```python
from build123d import *

# Parameters (mm, degrees)
SKETCH1_W                      = 260
SKETCH1_H                      = 250
BASE_FLANGE1_DEPTH             = 8
SKETCH2_R                      = 30
CUT_EXTRUDE1_DEPTH             = 10
EDGE_FLANGE1_STRIP_W           = 62
EDGE_FLANGE1_STRIP_H           = 8
EDGE_FLANGE1_STRIP_CUT_DEPTH   = 260
EDGE_FLANGE1_STRIP_2_W         = 62
EDGE_FLANGE1_STRIP_2_H         = 8
EDGE_FLANGE1_STRIP_CUT_2_DEPTH = 260
EDGE_FLANGE1_DEPTH             = 260
EDGE_FLANGE1_BEND_DEPTH        = 260
SKETCH9_R                      = 9
CUT_EXTRUDE2_DEPTH             = 10
SKETCH10_R                     = 8
CUT_EXTRUDE3_DEPTH             = 10
CIRPATTERN1_COUNT              = 4


# Sheet-metal steps are written as plain solids
with BuildPart() as part:
    # Sketch1 → Base-Flange1 (new body)
    with BuildSketch(Plane(origin=(0, 0, 0), x_dir=(0, 0, -1), z_dir=(1, 0, 0))):
        Rectangle(SKETCH1_W, SKETCH1_H)
    extrude(amount=-BASE_FLANGE1_DEPTH)

    # Sketch2 → Cut-Extrude1 (cut)
    with BuildSketch(Plane(origin=(0, 0, 0), x_dir=(0, 0, -1), z_dir=(1, 0, 0))):
        Circle(SKETCH2_R)
    extrude(amount=-CUT_EXTRUDE1_DEPTH, mode=Mode.SUBTRACT)

    # Edge-Flange1 strip (across the edge) → Edge-Flange1 strip cut (cut)
    with BuildSketch(Plane(origin=(0, 125, -130), x_dir=(0, -1, 0), z_dir=(0, 0, 1))):
        with Locations((-8, -4)):
            Rectangle(EDGE_FLANGE1_STRIP_W, EDGE_FLANGE1_STRIP_H)
    extrude(amount=EDGE_FLANGE1_STRIP_CUT_DEPTH, mode=Mode.SUBTRACT)

    # Edge-Flange1 strip 2 (across the edge) → Edge-Flange1 strip cut 2 (cut)
    with BuildSketch(Plane(origin=(0, -125, 130), x_dir=(0, 1, 0), z_dir=(0, 0, -1))):
        with Locations((-8, -4)):
            Rectangle(EDGE_FLANGE1_STRIP_2_W, EDGE_FLANGE1_STRIP_2_H)
    extrude(amount=EDGE_FLANGE1_STRIP_CUT_2_DEPTH, mode=Mode.SUBTRACT)

    # Edge-Flange1 section (across the edge) → Edge-Flange1 (add)
    with BuildSketch(Plane(origin=(0, 125, -130), x_dir=(0, -1, 0), z_dir=(0, 0, 1))):
        with BuildLine():
            Line((0, 15), (0, 32))
            Line((0, 32), (8, 32))
            Line((8, 32), (8, 15))
            ThreePointArc((8, 15), (12.393398282, 4.393398282), (23, 0))
            Line((23, 0), (23, -8))
            ThreePointArc((23, -8), (6.736544033, -1.263455967), (0, 15))
        make_face()
    extrude(amount=EDGE_FLANGE1_DEPTH)

    # Edge-Flange1 section 2 (across the edge) → Edge-Flange1 bend (add)
    with BuildSketch(Plane(origin=(0, -125, 130), x_dir=(0, 1, 0), z_dir=(0, 0, -1))):
        with BuildLine():
            Line((0, 15), (0, 32))
            Line((0, 32), (8, 32))
            Line((8, 32), (8, 15))
            ThreePointArc((8, 15), (12.393398282, 4.393398282), (23, 0))
            Line((23, 0), (23, -8))
            ThreePointArc((23, -8), (6.736544033, -1.263455967), (0, 15))
        make_face()
    extrude(amount=EDGE_FLANGE1_BEND_DEPTH)

    # Sketch9 → Cut-Extrude2 (cut)
    with BuildSketch(Plane(origin=(0, 0, 0), x_dir=(0, 0, -1), z_dir=(1, 0, 0))):
        with Locations((-105, -70)):
            Circle(SKETCH9_R)
        with Locations((-105, 70)):
            Circle(SKETCH9_R)
    cut_extrude2 = extrude(amount=-CUT_EXTRUDE2_DEPTH, mode=Mode.SUBTRACT)

    # Mirror1: Cut-Extrude2 across plane
    add(cut_extrude2.mirror(Plane.XY), mode=Mode.SUBTRACT)

    # Sketch10 → Cut-Extrude3 (cut)
    with BuildSketch(Plane.ZY.offset(8)):
        with Locations((55.5, 55.5)):
            Circle(SKETCH10_R)
    cut_extrude3 = extrude(amount=-CUT_EXTRUDE3_DEPTH, mode=Mode.SUBTRACT)

    # CirPattern1: Cut-Extrude3 ×4 about axis
    cirpattern1_axis = Axis((0, 0, 0), (1, 0, 0))
    for i in range(1, CIRPATTERN1_COUNT):
        add(cut_extrude3.rotate(cirpattern1_axis, i * 360 / CIRPATTERN1_COUNT), mode=Mode.SUBTRACT)


solid = part.part
```
Could you check a few things on this model? Use its own coordinates, in mm. A direction names the side the tool comes from. Round coordinates to 2 decimals unless told otherwise and drop trailing zeros. Loops run counter-clockwise (first coordinate to the right, second up) from the corner with the lowest first, then second, coordinate; pieces in that order, holes last. Notation, with made-up numbers: (31, 21) - (89, 21) arc R22 ccw to (89, 55) - close; hole circle Ø2 at (-15.5, -19.75). An arc over 180 degrees is marked (long way). Use CSV: the item, a comma, the result in double quotes.
Item 1: I need wall thicknesses on L1, parallel to Z at x = -3.75, y = -55.5; L2, parallel to Y at x = 30, z = -98.5; L3, parallel to Y at x = -6, z = 55. Which ranges of each line are inside material? Lowest first, please. Write a range as [from, to].
Here are the results:
L1,"z = [-130, -63.5], [-47.5, 47.5], [63.5, 130]"
L2,"y = [-125, -117], [117, 125]"
L3,"y = [-111.38, -63.48], [-47.52, 47.52], [63.48, 111.38]"
Item 2: For faces 1 (the flat face through (-1, 1, -130)), 2 (the cylindrical face through (4.51, 112.72, -1.82)), which set-ups out of +Z, -Z, +X, -X, +Y, -Y let a thin tool reach every point of the face, with its end or its side?
Here are the results:
face 1,"-Z, +X, -X, +Y, -Y"
face 2,"+Z, -Z, +X"
Item 3: If we section it at C-C on x = 18.5: List the corners of the cut face in (y, z) for me, then the cut area to 3 significant figures.
Here are the results:
outline,"(-125, -130) - (-117, -130) - (-117, 130) - (-125, 130) - close; (117, -130) - (125, -130) - (125, 130) - (117, 130) - close"
area,"4,160 mm²"
Item 4: If we mould it in two halves opening along Z, with no side actions, what happens to faces 3 (the cylindrical face through (-3.94, 1.32, 29.97)), 4 (the flat face through (-1, 1, 130)), 5 (the flat face through (32, -121, 2))? For each: pulls with the +Z half, pulls with the -Z half, needs draft (parallel to the pull), parting line crosses it, or undercut.
Here are the results:
face 3,"undercut"
face 4,"pulls with the +Z half"
face 5,"needs draft"
Item 5: Will these pins go through, and if not, where does the flat tip stop? pin 1 (4 mm diameter, centred on y = 63, z = 65, fed in from +X); pin 2 (23.5 mm diameter, centred on y = -70, z = -105, fed in from -X); pin 3 (3 mm diameter, centred on x = 4, z = 90, fed in from +Y).
Here are the results:
pin 1,"stops at x = 0"
pin 2,"stops at x = -8"
pin 3,"stops at y = 122.95"
Item 6: If we section it at B-B on y = 55.5: List the corners of the cut face in (x, z) for me, then the cut area to 3 significant figures.
Here are the results:
outline,"(-8, -130) - (0, -130) - (0, -63.5) - (-8, -63.5) - close; (-8, -47.5) - (0, -47.5) - (0, 47.5) - (-8, 47.5) - close; (-8, 63.5) - (0, 63.5) - (0, 130) - (-8, 130) - close"
area,"1,820 mm²"
Item 7: If we section it at D-D on y = 0: List the corners of the cut face in (x, z) for me.
Here are the results:
outline,"(-8, -130) - (0, -130) - (0, -30) - (-8, -30) - close; (-8, 30) - (0, 30) - (0, 130) - (-8, 130) - close"
Item 8: If we section it at A-A on z = 0: List the corners of the cut face in (x, y) for me.
Here are the results:
outline,"(-8, -102) arc R23 ccw to (15, -125) - (32, -125) - (32, -117) - (15, -117) arc R15 cw to (0, -102) - (0, -30) - (-8, -30) - close; (-8, 30) - (0, 30) - (0, 102) arc R15 cw to (15, 117) - (32, 117) - (32, 125) - (15, 125) arc R23 ccw to (-8, 102) - close"
